from build123d import *

# Parameters (mm, degrees)
IZIM1_W                     = 40
IZIM1_H                     = 25
IZIM1_R                     = 1.25
Y_KSEKLIK_EKSTR_ZYON1_DEPTH = 2.5


with BuildPart() as part:
    # Çizim1 → Yükseklik-Ekstrüzyon1 (new body)
    with BuildSketch(Plane.YZ):
        with Locations((20, 12.5)):
            Rectangle(IZIM1_W, IZIM1_H)
        with Locations(Location((3, 22, 0), (0, 0, 270))):
            Circle(IZIM1_R, mode=Mode.SUBTRACT)
        with Locations(Location((13.7, 22, 0), (0, 0, 270))):
            Circle(IZIM1_R, mode=Mode.SUBTRACT)
        with Locations(Location((24.4, 22, 0), (0, 0, 270))):
            Circle(IZIM1_R, mode=Mode.SUBTRACT)
        with Locations(Location((35.1, 22, 0), (0, 0, 270))):
            Circle(IZIM1_R, mode=Mode.SUBTRACT)
    extrude(amount=Y_KSEKLIK_EKSTR_ZYON1_DEPTH)


solid = part.part
Verification items for the finished model (mm, model axes). Round coordinates to 2 decimals unless told otherwise and drop trailing zeros. Loops run counter-clockwise (first coordinate to the right, second up) from the corner with the lowest first, then second, coordinate; pieces in that order, holes last. Notation, with made-up numbers: (83, -16) - (137, -16) arc R31 ccw to (137, 16) - close; hole circle Ø3 at (-23.5, 87). An arc over 180 degrees is marked (long way). Answer in a Markdown table with one row per item. Add a question column.
Q1. Material ranges on line 1 (Y direction, x = 1.7, z = 22); line 2 (Z direction, x = 1.55, y = 34), recorded low to high.
Q2. Gauge pin test, flat end, axial feed: pin 1 (1.5 mm diameter, centred on y = 24.4, z = 22, fed in from -X). Record the tip position at first contact, or that the pin passes through.
Q3. Release check for a two-part mould opening along Z. For faces 1 (the face through (1, 20, 25)), 2 (the face through (1, 20, 0)), 3 (the face through (1.232, 25.454, 21.328)), 4 (the face through (1, 40, 12)) record: pulls with the +Z half, pulls with the -Z half, needs draft (parallel to the pull), parting line crosses it, or undercut.
Q4. Section check B-B on y = 13.7. Enter the section's corners in (x, z), plus the area to 4 significant figures.
Q5. Section check C-C on y = 24. Enter the section's corners in (x, z).
Q6. Section check A-A on x = 1.9. Enter the section's corners in (y, z).
Found:
| question | item | result |
|---|---|---|
| 1 | line 1 | y = 0 to 1.75, 4.25 to 12.45, 14.95 to 23.15, 25.65 to 33.85, 36.35 to 40 |
| 1 | line 2 | z = 0 to 21.41, 22.59 to 25 |
| 2 | pin 1 | passes through |
| 3 | face 1 | pulls with the +Z half |
| 3 | face 2 | pulls with the -Z half |
| 3 | face 3 | undercut |
| 3 | face 4 | needs draft |
| 4 | outline | (0, 0) - (2.5, 0) - (2.5, 20.75) - (0, 20.75) - close; (0, 23.25) - (2.5, 23.25) - (2.5, 25) - (0, 25) - close |
| 4 | area | 56.25 mm² |
| 5 | outline | (0, 0) - (2.5, 0) - (2.5, 20.82) - (0, 20.82) - close; (0, 23.18) - (2.5, 23.18) - (2.5, 25) - (0, 25) - close |
| 6 | outline | (0, 0) - (40, 0) - (40, 25) - (0, 25) - close; hole circle Ø2.5 at (3, 22); hole circle Ø2.5 at (13.7, 22); hole circle Ø2.5 at (24.4, 22); hole circle Ø2.5 at (35.1, 22) |
